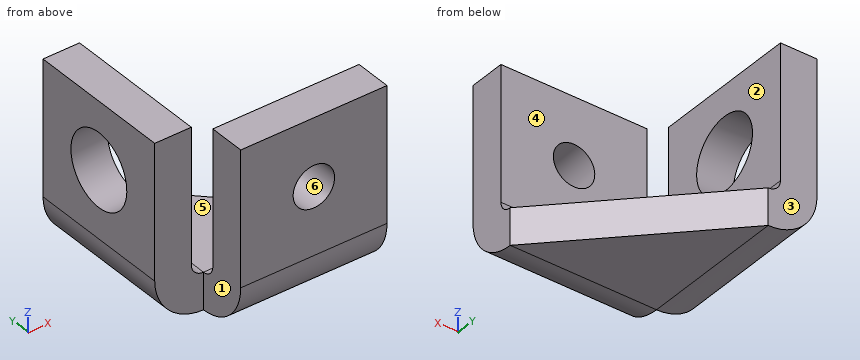
Autodesk Inventor part; units mm, degrees
ref_plane "YZ Plane" through (0, 0, 0) normal (1, 0, 0) x (0, 1, 0)
ref_plane "XZ Plane" through (0, 0, 0) normal (0, 1, 0) x (-1, 0, 0)
ref_plane "XY Plane" through (0, 0, 0) normal (0, 0, 1) x (1, 0, 0)
sketch "Sketch1" plane through (0, 0, 0) normal (0, 0, 1) x (1, 0, 0)
  line L0 (0, 0) -> (16, 0)
  line L1 (16, 0) -> (16, 16)
  line L2 (16, 16) -> (0, 16)
  line L3 (0, 16) -> (0, 0)
  line L4 (4, 16) -> (16, 4)
  dimension "d0" = 45
  dimension "d1" = 16
  dimension "d2" = 16
  dimension "d3" = 4
extrude "Extrusion1" add sketch "Sketch1" along normal blind 3 contours L3 L2 L4 L1 L0
sketch "Sketch2" plane through (0, 0, 3) normal (0, 0, 1) x (1, 0, 0)
  line L0 (0, 0) -> (16, 0)
  line L1 (16, 0) -> (16, 4)
  line L2 (16, 4) -> (4, 16)
  line L3 (4, 16) -> (0, 16)
  line L4 (0, 16) -> (0, 0)
  line L5 (4, 16) -> (0, 16)
  line L6 (0, 0) -> (3, 0)
  line L7 (3, 0) -> (3, 16)
  line L8 (3, 16) -> (0, 16)
  line L9 (0, 16) -> (0, 0)
  line L10 (16, 3) -> (0, 3)
  line L11 (0, 3) -> (0, 0)
  line L12 (0, 0) -> (16, 0)
  line L13 (16, 0) -> (16, 3)
  dimension "d20" = 3
  dimension "d21" = 3
extrude "Extrusion2" add sketch "Sketch2" along normal blind 12 contours L4 L10 L7 L0 | L7 L10 L1 L0 | L4 L3 L7 L10
sketch "Sketch6" plane through (0, 0, 15) normal (0, 0, 1) x (1, 0, 0)
  line L0 (0, 0) -> (4, 0)
  line L1 (4, 0) -> (4, 4)
  line L2 (4, 4) -> (0, 4)
  line L3 (0, 4) -> (0, 0)
  line L4 (3, 3) -> (3, 16)
  line L5 (16, 3) -> (3, 3)
  dimension "d22" = 1
  dimension "d23" = 1
extrude "Extrusion5" cut sketch "Sketch6" against normal through all
fillet "Fillet1" radius 1 2 edges at (3, 10, 3) (10, 3, 3)
fillet "Fillet2" radius 4 2 edges at (0, 10, 0) (10, 0, 0)
sketch "Sketch7" plane through (3, 4, 15) normal (1, 0, 0) x (0, 0, -1)
  line L0 (0, 0) -> (0, 12)
  line L1 (11, 12) -> (0, 12)
  point P0 (15, -4)
  point P1 (5.5, 6)
  point P2 (0, 6)
  point P3 (5.5, 12)
hole "Hole1" at (3, 10, 9.5) direction (-1, 0, 0) diameter 6 end through all
sketch "Sketch8" plane through (4, 3, 15) normal (0, 1, 0) x (1, 0, 0)
  line L0 (0, 11) -> (0, 0)
  line L1 (12, 0) -> (0, 0)
  point P0 (-4, 15)
  point P1 (6, 5.5)
  point P2 (0, 5.5)
  point P3 (6, 0)
hole "Hole2" at (10, 3, 9.5) direction (0, -1, 0) diameter 3.4 end through all
equation "\"d2\" = d1"
equation "\"d21\" = d20"
equation "\"d23\" = d22"
properties part number "Top_Cable End" material "Aluminum 6061"
Verification items for the finished model (mm, model axes). Face numbers are marked on the shaded views. A direction names the side the tool comes from. Coordinates: 2 decimals unless noted, no trailing zeros. Order: outer loops, then holes, each group sorted by start corner. A loop starts at its lowest first (then second) coordinate and runs counter-clockwise, first axis right, second up. Notation, with made-up numbers: M 20,64 L 34,64 A15 ccw 34,74 Z; hole C 38.25,-4 d11. An arc over 180 degrees is marked long. Return JSON: item names as keys, results as strings.
1) Gauge pin test, flat ends, axial feed: pin 1 (1.5 mm diameter, centred on x = 9.5, z = 10, fed in from +Y); pin 2 (2 mm diameter, centred on y = 7.5, z = 4.5, fed in from +X); pin 3 (3 mm diameter, centred on y = 2, z = 5.5, fed in from -X); pin 4 (9 mm diameter, centred on x = 8.5, z = 9, fed in from +Y). Record the tip position at first contact, or that the pin passes through.
Answer list:
{"pin 1": "through", "pin 2": "x = 3.13", "pin 3": "x = 4", "pin 4": "y = 3"}
2) Cross-section at A-A, the plane y = 10. Record the boundary of the cut face in (x, z).
Answer list:
{"outline": "M 0,4 A4 ccw 4,0 L 10,0 L 10,3 L 4,3 A1 cw 3,4 L 3,6.5 L 0,6.5 Z; M 0,12.5 L 3,12.5 L 3,15 L 0,15 Z"}
3) Access from +Z, -Z, +X, -X, +Y, -Y to the whole of each face (thin tool, end or side, straight path). Record for the marked faces 1, 2 and 3.
Answer list:
{"face 1": "+Z, -Z, -X, -Y", "face 2": "+Z, +X, +Y, -Y", "face 3": "+Z, -Z, +X, -X, +Y"}
4) Cross-section at D-D, the plane z = 5.25. Record the boundary of the cut face in (x, y).
Answer list:
{"outline": "M 0,4 L 3,4 L 3,16 L 0,16 Z; M 4,0 L 16,0 L 16,3 L 4,3 Z"}
5) Cross-section at B-B, the plane z = 9.5. Record the boundary of the cut face in (x, y).
Answer list:
{"outline": "M 0,4 L 3,4 L 3,7 L 0,7 Z; M 0,13 L 3,13 L 3,16 L 0,16 Z; M 4,0 L 8.3,0 L 8.3,3 L 4,3 Z; M 11.7,0 L 16,0 L 16,3 L 11.7,3 Z"}
6) Thickness scan on L1, parallel to X at y = 1, z = 9.5; L2, parallel to Y at x = 2.25, z = 9.5; L3, parallel to X at y = 14.25, z = 6. Record the ranges inside material, lowest first. Write a range as [from, to].
Answer list:
{"L1": "[4, 8.3], [11.7, 16]", "L2": "[4, 7], [13, 16]", "L3": "[0, 3]"}
7) Release check for a two-part mould opening along Z. For the marked faces 4, 5 and 6 record: +Z half, -Z half, draft (parallel to the pull), parting line (faces both ways), or undercut.
Answer list:
{"face 4": "draft", "face 5": "+Z half", "face 6": "undercut"}
8) Cross-section at C-C, the plane x = 10. Record the boundary of the cut face in (y, z), and give its area (3 significant figures).
Answer list:
{"outline": "M 0,4 A4 ccw 4,0 L 10,0 L 10,3 L 4,3 A1 cw 3,4 L 3,7.8 L 0,7.8 Z; M 0,11.2 L 3,11.2 L 3,15 L 0,15 Z", "area": "52.6 mm2"}
